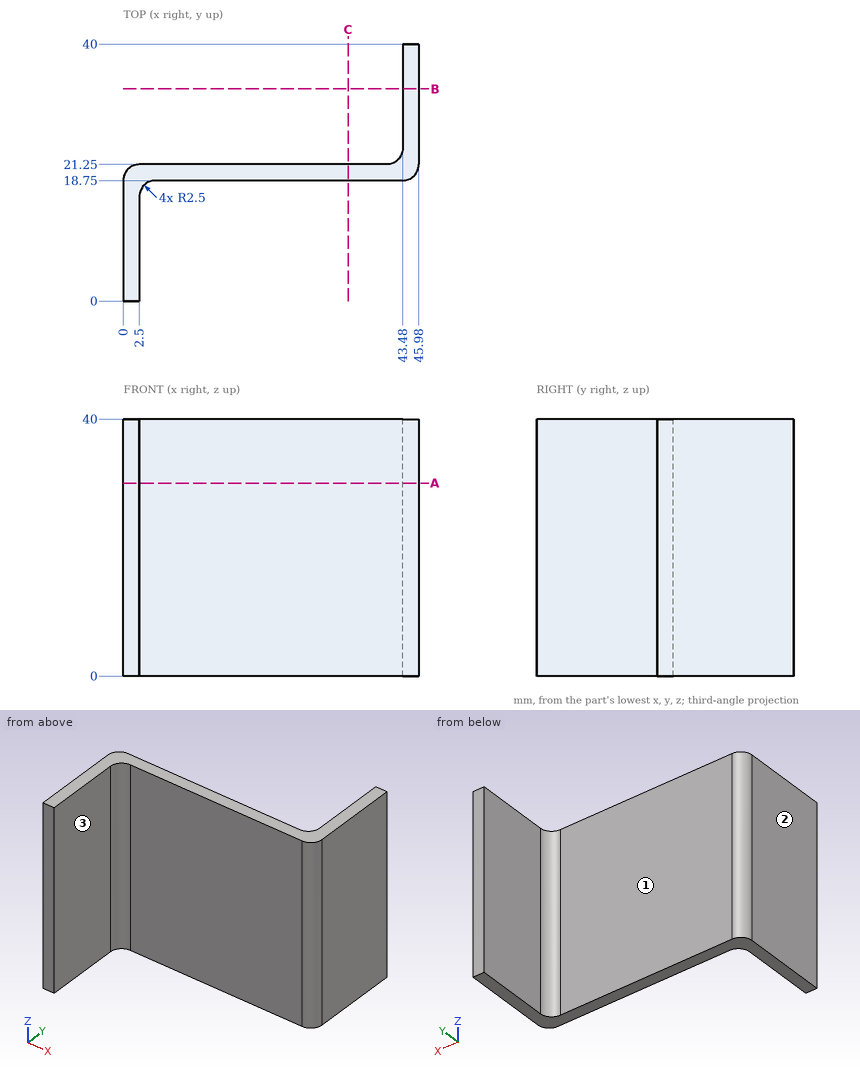
Source: three-view drawing plus pictorial views. Frame: mm from the lowest corner of the part. A direction names the side the tool comes from. Coordinates: 2 decimals unless noted, no trailing zeros. Order: outer loops, then holes, each group sorted by start corner. A loop starts at its lowest first (then second) coordinate and runs counter-clockwise, first axis right, second up.
1) Ray query, probe 1 along Y at (x, z) = (8.5, 21); probe 2 along X at (y, z) = (24.5, 38); probe 3 along X at (y, z) = (2, 19.5). Return the intervals inside material, ascending.
Result sheet:
probe 1: y = 18.75 to 21.25
probe 2: x = 43.48 to 45.98
probe 3: x = 0 to 2.5
2) Section A-A (z = 30). Return loops of the section in (x, y), then the cut area to 3 significant figures.
Result sheet:
outline: (0, 0) - (2.5, 0) - (2.5, 16.25) arc R2.5 cw to (5, 18.75) - (43.48, 18.75) arc R2.5 ccw to (45.98, 21.25) - (45.98, 40) - (43.48, 40) - (43.48, 23.75) arc R2.5 cw to (40.98, 21.25) - (2.5, 21.25) arc R2.5 ccw to (0, 18.75) - close
area: 209 mm2
3) First-contact query: P1, Ø1.5, axis at x = 18, z = 18.5, coming from the +Y side; P2, Ø4, axis at y = 34, z = 22.5, coming from the -X side; P3, Ø5, axis at y = 7.5, z = 12.5, coming from the +X side; P4, Ø10, axis at x = 12, y = 24, coming from the +Z side. Flat tips, straight axial feed; report the tip coordinate or a pass-through.
Result sheet:
P1: stops at y = 21.25
P2: stops at x = 43.48
P3: stops at x = 2.5
P4: stops at z = 40
4) Set-up query: the marked faces 1, 2 and 3. Return all of +Z, -Z, +X, -X, +Y, -Y with unobstructed straight access to the full face (end or side cutting, diameter ignored); none if empty.
Result sheet:
face 1: +Z, -Z, -X, +Y
face 2: +Z, -Z, -X, +Y, -Y
face 3: +Z, -Z, +X, -Y
5) Section B-B (y = 33). Return loops of the section in (x, z).
Result sheet:
outline: (43.48, 0) - (45.98, 0) - (45.98, 40) - (43.48, 40) - close
6) Section C-C (x = 35). Return loops of the section in (y, z).
Result sheet:
outline: (18.75, 0) - (21.25, 0) - (21.25, 40) - (18.75, 40) - close
